from build123d import *

# Parameters (mm, degrees)
F0_W     = 37.35
F0_H     = 77
F0_R     = 2
F0_W_2   = 14.55
F0_H_2   = 26.48
F1_DEPTH = 2
F2_R     = 3
F3_R     = 1


# Not quite as in the source:
# - a feature of the source that left no trace in its solid (it failed there, or was rolled back) is left out


with BuildPart() as f1:
    # F0 (on Top) → F1 (new body)
    with BuildSketch(Plane.XY):
        Rectangle(F0_W, F0_H)
        with Locations((-13.105, -35.5)):
            Circle(F0_R, mode=Mode.SUBTRACT)
        with Locations((-8.35, -19.26)):
            Rectangle(F0_W_2, F0_H_2, mode=Mode.SUBTRACT)
        with Locations((10.175, -27.3)):
            Circle(F0_R, mode=Mode.SUBTRACT)
        with Locations((10.175, -10.5)):
            Circle(F0_R, mode=Mode.SUBTRACT)
        with Locations((-15.675, 35.5)):
            Circle(F0_R, mode=Mode.SUBTRACT)
        with Locations((10.175, 5.72)):
            Circle(F0_R, mode=Mode.SUBTRACT)
        with Locations((10.175, 23.25)):
            Circle(F0_R, mode=Mode.SUBTRACT)
    extrude(amount=F1_DEPTH)

    # F2
    f2_edges = [f1.edges().sort_by_distance(p)[0] for p in [
        (-1.075, -6.02, 1),
        (-1.075, -32.5, 1),
        (-15.625, -32.5, 1),
        (-15.625, -6.02, 1),
    ]]
    fillet(f2_edges, radius=F2_R)

    # F3
    f3_edges = [f1.edges().sort_by_distance(p)[0] for p in [
        (-18.675, -38.5, 1),
        (18.675, -38.5, 1),
        (18.675, 38.5, 1),
        (-18.675, 38.5, 1),
    ]]
    fillet(f3_edges, radius=F3_R)


solid = f1.part
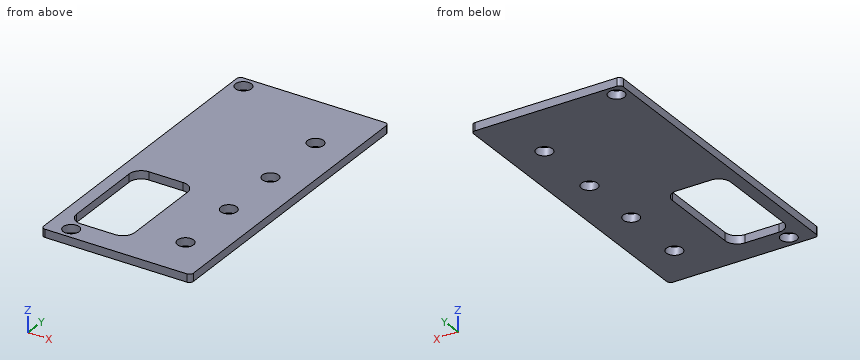
Geometry: final body of the model. Coordinates: model frame, mm. Round coordinates to 2 decimals unless told otherwise and drop trailing zeros. Loops run counter-clockwise (first coordinate to the right, second up) from the corner with the lowest first, then second, coordinate; pieces in that order, holes last. Notation, with made-up numbers: (69.25, 36.5) -> (91.25, 36.5) arc R31 cw to (91.25, 66.5) -> close; hole circle Ø6 at (3.25, -0.75). An arc over 180 degrees is marked (long way). One line per question, with ' | ' between items. Start each with the question number.
1. Section C-C on y = -27.3. Output: boundary loops of the cut face in (x, z) (3 decimals), and give its area (3 significant figures).
2. Contact query for a flat-ended pin moving along its axis: pin 1 (2.5 mm diameter, centred on x = -13.105, y = -35.5, fed in from +Z). Output: stop coordinate, or through.
3. Section D-D on x = -2. Output: boundary loops of the cut face in (y, z).
4. Line query: line 1 along Y through (x, z) = (-11, 1.45); line 2 along X through (y, z) = (-22, 0.75) (3 decimals); line 3 along Y through (x, z) = (-11.5, 0.3). Output: solid intervals per line, ascending. Write a range as [from, to].
5. Section B-B on z = 1.7. Output: boundary loops of the cut face in (x, y) (3 decimals).
6. Section A-A on y = -17. Output: boundary loops of the cut face in (x, z) (3 decimals).
Returned:
1) outline: (-18.675, 0) -> (-15.625, 0) -> (-15.625, 2) -> (-18.675, 2) -> close; (-1.075, 0) -> (8.175, 0) -> (8.175, 2) -> (-1.075, 2) -> close; (12.175, 0) -> (18.675, 0) -> (18.675, 2) -> (12.175, 2) -> close | area: 37.6 mm2
2) pin 1: passes through
3) outline: (-38.5, 0) -> (-31.67, 0) -> (-31.67, 2) -> (-38.5, 2) -> close; (-6.85, 0) -> (38.5, 0) -> (38.5, 2) -> (-6.85, 2) -> close
4) line 1: y = [-38.5, -32.5], [-6.02, 38.5] | line 2: x = [-18.675, -15.625], [-1.075, 18.675] | line 3: y = [-38.5, -36.69], [-34.31, -32.5], [-6.02, 38.5]
5) outline: (-18.675, -37.5) arc R1 ccw to (-17.675, -38.5) -> (17.675, -38.5) arc R1 ccw to (18.675, -37.5) -> (18.675, 37.5) arc R1 ccw to (17.675, 38.5) -> (-17.675, 38.5) arc R1 ccw to (-18.675, 37.5) -> close; hole circle Ø4 at (-15.675, 35.5); hole (-15.625, -29.5) arc R3 ccw to (-12.625, -32.5) -> (-4.075, -32.5) arc R3 ccw to (-1.075, -29.5) -> (-1.075, -9.02) arc R3 ccw to (-4.075, -6.02) -> (-12.625, -6.02) arc R3 ccw to (-15.625, -9.02) -> close; hole circle Ø4 at (-13.105, -35.5); hole circle Ø4 at (10.175, -27.3); hole circle Ø4 at (10.175, -10.5); hole circle Ø4 at (10.175, 5.72); hole circle Ø4 at (10.175, 23.25)
6) outline: (-18.675, 0) -> (-15.625, 0) -> (-15.625, 2) -> (-18.675, 2) -> close; (-1.075, 0) -> (18.675, 0) -> (18.675, 2) -> (-1.075, 2) -> close
